Input: part model. Units: mm. Frame: model coordinates. A direction names the side the tool comes from. Give positions to 0.01 mm unless a question says otherwise; leave off trailing zeros. Write each loop counter-clockwise with the first axis right and the second up, starting at its lowest first coordinate (ties: lowest second). Pieces come first, ordered by that corner, then holes. Notation, with made-up numbers: (83.5, 59.25) -> (133.5, 59.25) arc R34 ccw to (133.5, 91.25) -> close; hole circle Ø3 at (63.5, -21.5). An arc over 180 degrees is marked (long way). Return JSON: item names as keys, results as strings. Group by question number.
Item 1: Section D-D, the plane y = -2.5. Return loops of the section in (x, z).
Item 2: Pin query (flat end, axial travel): P1, Ø6, axis at x = 2, y = 3.5, coming from the -Z side; P2, Ø1, axis at y = 5, z = -18.5, coming from the +X side; P3, Ø2, axis at y = 6, z = -1.5, coming from the -X side. Return the tip coordinate at first contact, or that it passes through.
Item 3: Mould query, pull axis Z, two halves, no side actions, for faces 4 (the face through (2.92, 10.85, -19.17)), 5 (the face through (-5.3, -4, -12.7)), 6 (the face through (4.144, 21.507, -4.923)). Classes: released by +Z, released by -Z, zero draft, split by the parting line, or undercut.
Item 4: Section C-C, the plane y = 15.25. Return loops of the section in (x, z), then the cut area to 3 significant figures.
Item 5: Line query: line 1 (X direction, y = -1.5, z = -9.75); line 2 (Y direction, x = 1.5, z = -2.5); line 3 (Y direction, x = -2.5, z = -21.5). Output: solid intervals per line, ascending. Write a range as [from, to].
Item 6: Section B-B, the plane x = -18. Return loops of the section in (y, z).
Item 7: Section A-A, the plane z = -17.5. Return loops of the section in (x, y).
Item 8: Set-up query: faces 1 (the face through (-2, 22, 2)), 2 (the face through (-0.726, 21.507, -11.813)), 3 (the face through (-10.58, -1.97, -7.28)). Return all of +Z, -Z, +X, -X, +Y, -Y with unobstructed straight access to the full face (end or side cutting, diameter ignored); none if empty.
Autodesk Inventor part; units mm, degrees
ref_plane "YZ Plane" through (0, 0, 0) normal (1, 0, 0) x (0, 1, 0)
ref_plane "XZ Plane" through (0, 0, 0) normal (0, 1, 0) x (-1, 0, 0)
ref_plane "XY Plane" through (0, 0, 0) normal (0, 0, 1) x (1, 0, 0)
sketch "Эскиз1" plane through (0, 0, 0) normal (0, 1, 0) x (-1, 0, 0)
  circle A0 centre (7.4029, -9.7102) radius 14
  point P0 (0, 0)
  dimension "d0" = 28
extrude "Выдавливание1" add sketch "Эскиз1" along normal blind 22
sketch "Эскиз2" plane through (-7.4029, 22, -9.7102) normal (0, 1, 0) x (1, 0, 0)
  circle A0 centre (0, 0) radius 12.5
  circle A1 centre (0, 0) radius 7
  point P0 (7.4029, -9.7102)
  dimension "d6" = 25
  dimension "d7" = 14
extrude "Выдавливание2" cut sketch "Эскиз2" against normal blind 1
sketch "Эскиз3" plane through (-7.4029, 0, -9.7102) normal (0, -1, 0) x (1, 0, 0)
  circle A0 centre (0, 0) radius 4
  circle A1 centre (0, 0) radius 3.5
  point P0 (7.4029, 9.7102)
  dimension "d8" = 8
  dimension "d9" = 7
extrude "Выдавливание3" add sketch "Эскиз3" along normal blind 4
properties part number "магнит" material "Титан"
Answer below:
{
 "1": {"outline": "circle Ø8 at (-7.4, -9.71); hole circle Ø7 at (-7.4, -9.71)"},
 "2": {"P1": "stops at z = -22.16", "P2": "stops at x = 3.88", "P3": "stops at x = -19.4"},
 "3": {"face 4": "split by the parting line", "face 5": "zero draft", "face 6": "undercut"},
 "4": {"outline": "circle Ø28 at (-7.4, -9.71)", "area": "616 mm2"},
 "5": {"line 1": "x = [-11.4, -10.9], [-3.9, -3.4]", "line 2": "y = [0, 21]", "line 3": "y = [0, 22]"},
 "6": {"outline": "(0, -18.86) -> (22, -18.86) -> (22, -16.34) -> (21, -16.34) -> (21, -3.08) -> (22, -3.08) -> (22, -0.56) -> (0, -0.56) -> close"},
 "7": {"outline": "(-19.04, 0) -> (4.23, 0) -> (4.23, 22) -> (2.37, 22) -> (2.37, 21) -> (-17.18, 21) -> (-17.18, 22) -> (-19.04, 22) -> close"},
 "8": {"face 1": "+Z, -Z, +X, -X, +Y", "face 2": "+Y", "face 3": "-Y"}
}
